Can you work these out from the model? Positions are in its coordinate system, mm. A direction names the side the tool comes from. Coordinates: 2 decimals unless noted, no trailing zeros. Order: outer loops, then holes, each group sorted by start corner. A loop starts at its lowest first (then second) coordinate and runs counter-clockwise, first axis right, second up.
```python
from build123d import *

# Parameters (mm, degrees)
SKETCH1_R            = 27.5
SKETCH1_W            = 37
SKETCH1_H            = 37
BOSS_EXTRUDE1_DEPTH  = 6
SKETCH1_3_W          = 37
SKETCH1_3_H          = 37
SKETCH1_3_W_2        = 35
SKETCH1_3_H_2        = 35
BOSS_EXTRUDE2_DEPTH  = 1
M2_CLEARANCE_HOLE1_D = 2.6
M2_CLEARANCE_HOLE2_D = 2.4
CUT_EXTRUDE3_DEPTH   = 0.8


with BuildPart() as part:
    # Sketch1 → Boss-Extrude1 (new body)
    with BuildSketch(Plane.XY):
        Circle(SKETCH1_R)
        Rectangle(SKETCH1_W, SKETCH1_H, mode=Mode.SUBTRACT)
    extrude(amount=BOSS_EXTRUDE1_DEPTH)

    # Sketch1_3 → Boss-Extrude2 (add)
    # profile 1 of 2: a face of its own
    with BuildSketch(Plane.XY):
        Rectangle(SKETCH1_3_W, SKETCH1_3_H)
        Rectangle(SKETCH1_3_W_2, SKETCH1_3_H_2, mode=Mode.SUBTRACT)
    # profile 2 of 2: a face of its own
    with BuildSketch(Plane.XY):
        Rectangle(SKETCH1_3_W_2, SKETCH1_3_H_2)
    extrude(amount=BOSS_EXTRUDE2_DEPTH)

    # Sketch2 → Revolve1 (revolve)
    with BuildSketch(Plane(origin=(0, 0, 0), x_dir=(1, 0, 0), z_dir=(0, 1, 0)), mode=Mode.PRIVATE) as revolve1_sk:
        with BuildLine():
            Line((0, 6.5), (0, 0))
            Line((0, 0), (-6.5, 0))
            ThreePointArc((-6.5, 0), (-4.596194078, 4.596194078), (0, 6.5))
        make_face()
    revolve(revolve1_sk.sketch.rotate(Axis((0, 0, -15), (0, 0, 1)), 180), axis=Axis((0, 0, -15), (0, 0, 1)))

    # M2 Clearance Hole1 (through all)
    with Locations(Plane.XY.offset(6)):
        with Locations((-21, 0), (14, -21), (14, 21)):
            Hole(M2_CLEARANCE_HOLE1_D / 2)

    # M2 Clearance Hole2 (through all)
    with Locations(Plane(origin=(0, 20, 0), x_dir=(-1, 0, 0), z_dir=(0, 0, -1))):
        with Locations((0, 0), (0, -40)):
            Hole(M2_CLEARANCE_HOLE2_D / 2)

    # Sketch5 → Cut-Extrude3 (cut)
    with BuildSketch(Plane.XY):
        Polygon((0, 17.401923789), (2.25, 18.700961894), (2.25, 21.299038106), (0, 22.598076211), (-2.25, 21.299038106), (-2.25, 18.700961894), align=None)
        Polygon((-2.25, -18.700961894), (0, -17.401923789), (2.25, -18.700961894), (2.25, -21.299038106), (0, -22.598076211), (-2.25, -21.299038106), align=None)
    extrude(amount=CUT_EXTRUDE3_DEPTH, mode=Mode.SUBTRACT)


solid = part.part
```
1. Imagine slicing it at A-A on z = 4.25. Please give me the cut outline in (x, y), then the cut area to 3 significant figures.
Completed:
outline: circle Ø55 at (0, 0); hole circle Ø2.6 at (-21, 0); hole (-18.5, -18.5) - (18.5, -18.5) - (18.5, 18.5) - (-18.5, 18.5) - close; hole circle Ø2.4 at (0, -20); hole circle Ø2.4 at (0, 20); hole circle Ø2.6 at (14, -21); hole circle Ø2.6 at (14, 21)
area: 982 mm2
2. I'm going to push flat-ended pins straight in: pin 1 (5.5 mm diameter, centred on x = 8, z = 4.5, fed in from -Y); pin 2 (1.3 mm diameter, centred on x = 0, y = 19, fed in from -Z); pin 3 (2 mm diameter, centred on x = -5.5, z = 2, fed in from +Y). Where does each tip first touch, or does it pass through?
Completed:
pin 1: stops at y = -26.99
pin 2: stops at z = 0.8
pin 3: stops at y = 27.13
3. Please list where these lines run through material, in increasing order: probe 1 along Y at (x, z) = (0, 2.85); probe 2 along Z at (x, y) = (-23.5, -7); probe 3 along Z at (x, y) = (7.5, 3.5).
Completed:
probe 1: y = -27.5 to -21.2, -18.8 to -18.5, 18.5 to 18.8, 21.2 to 27.5
probe 2: z = 0 to 6
probe 3: z = 0 to 1
4. On a 3-axis mill with a long thin cutter (end or side, diameter ignored), from which of +Z, -Z, +X, -X, +Y, -Y can I reach the whole of each face in a straight line? I mean faces 1 (the flat face through (-1.109, -21.958, 0.394)), 2 (the flat face through (0, 0, 1)), 3 (the cylindrical face through (-0.26, -21.17, 3.44)). Say none if no direction works.
Completed:
face 1: -Z
face 2: +Z
face 3: +Z, -Z
5. Imagine slicing it at C-C on x = -12. Please give me the cut outline in (y, z).
Completed:
outline: (-24.74, 0) - (24.74, 0) - (24.74, 6) - (18.5, 6) - (18.5, 1) - (-18.5, 1) - (-18.5, 6) - (-24.74, 6) - close
6. Thinking about a two-plate mould opening in Y: for faces 4 (the flat face through (6, -6, 0)), 5 (the cylindrical face through (-0.26, 18.83, 3.44)), which applies, pulls with the +Y half, pulls with the -Y half, needs draft (parallel to the pull), parting line crosses it, or undercut?
Completed:
face 4: needs draft
face 5: undercut
7. Imagine slicing it at B-B on x = -21. Please give me the cut outline in (y, z), then the cut area to 3 significant figures.
Completed:
outline: (-17.76, 0) - (-1.3, 0) - (-1.3, 6) - (-17.76, 6) - close; (1.3, 0) - (17.76, 0) - (17.76, 6) - (1.3, 6) - close
area: 197 mm2
8. Imagine slicing it at D-D on y = 3.5. Please give me the cut outline in (x, z).
Completed:
outline: (-27.28, 0) - (-5.48, 0) arc R5.48 ccw to (5.48, 0) - (27.28, 0) - (27.28, 6) - (18.5, 6) - (18.5, 1) - (-18.5, 1) - (-18.5, 6) - (-27.28, 6) - close
